from build123d import *

# Parameters (mm, degrees)
IZIM1_R                     = 3.787969925
Y_KSEKLIK_EKSTR_ZYON1_DEPTH = 3.7


with BuildPart() as part:
    # Çizim1 → Yükseklik-Ekstrüzyon1 (new body)
    with BuildSketch(Plane.XY):
        with BuildLine():
            Line((-7.697744361, -49), (-7.697744361, 49))
            ThreePointArc((-7.697744361, 49), (0, 56.697744361), (7.697744361, 49))
            Line((7.697744361, 49), (7.697744361, -49))
            ThreePointArc((7.697744361, -49), (0, -56.697744361), (-7.697744361, -49))
        make_face()
        with Locations((0, -45)):
            Circle(IZIM1_R, mode=Mode.SUBTRACT)
        with Locations(Location((0, 45, 0), (0, 0, 180))):
            Circle(IZIM1_R, mode=Mode.SUBTRACT)
    extrude(amount=Y_KSEKLIK_EKSTR_ZYON1_DEPTH)


solid = part.part
Model file for the job. Use its own axes, mm. Give positions to 0.01 mm unless a question says otherwise; leave off trailing zeros. Loops run counter-clockwise (first coordinate to the right, second up) from the corner with the lowest first, then second, coordinate; pieces in that order, holes last.
Item 1: Slice it at B-B (z = 2). Write the cut outline in (x, y).
Check values:
outline: (-7.7, -49) arc R7.7 ccw to (7.7, -49) - (7.7, 49) arc R7.7 ccw to (-7.7, 49) - close; hole circle Ø7.58 at (0, -45); hole circle Ø7.58 at (0, 45)
Item 2: Drop flat-ended pins along their axis: P1, Ø2, axis at x = 5.5, z = 3, coming from the -Y side; P2, Ø1, axis at x = 5.5, z = 0.5, coming from the +Y side. Give the stop position or say it passes through.
Check values:
P1: stops at y = -55.25
P2: stops at y = 54.85
Item 3: Mould opens along Y. For faces 1 (the face through (0.169, -56.696, 1.824)), 2 (the face through (0.493, 41.244, 1.824)), 3 (the face through (7.698, 1, 2)) say: +Y half, -Y half, draft (parallel to the pull), parting line (faces both ways), or undercut.
Check values:
face 1: -Y half
face 2: undercut
face 3: draft
Item 4: Drill centre lines: line 1 along Y through (x, z) = (0, 1.1); line 2 along X through (y, z) = (45, 1.45); line 3 along Y through (x, z) = (1.75, 3.45). Where is each one in solid material? Low to high.
Check values:
line 1: y = -56.7 to -48.79, -41.21 to 41.21, 48.79 to 56.7
line 2: x = -7.7 to -3.79, 3.79 to 7.7
line 3: y = -56.5 to -48.36, -41.64 to 41.64, 48.36 to 56.5
Item 5: Slice it at A-A (y = 45). Write the cut outline in (x, z), plus the area to 3 significant figures.
Check values:
outline: (-7.7, 0) - (-3.79, 0) - (-3.79, 3.7) - (-7.7, 3.7) - close; (3.79, 0) - (7.7, 0) - (7.7, 3.7) - (3.79, 3.7) - close
area: 28.9 mm2
Item 6: Slice it at C-C (x = 6.25). Write the cut outline in (y, z).
Check values:
outline: (-53.49, 0) - (53.49, 0) - (53.49, 3.7) - (-53.49, 3.7) - close
